from build123d import *

# Parameters (mm, degrees)
SKETCH1_R           = 1.4
BOSS_EXTRUDE1_DEPTH = 3
SKETCH2_R           = 1.4
BOSS_EXTRUDE2_DEPTH = 3
SKETCH3_W           = 32
SKETCH3_H           = 35.2
BOSS_EXTRUDE3_DEPTH = 3


with BuildPart() as part:
    # Sketch1 → Boss-Extrude1 (new body)
    with BuildSketch(Plane(origin=(0, 0, 0), x_dir=(1, 0, 0), z_dir=(0, 1, 0))):
        Polygon((-16, 24), (-16, -6), (16, -6), (16, 24), (10, 24), (10, 0), (-10, 0), (-10, 24), align=None)
        with Locations(Location((-8, -3.307692308, 0), (0, 0, 270))):
            Circle(SKETCH1_R, mode=Mode.SUBTRACT)
        with Locations(Location((8, -3.307692308, 0), (0, 0, 90))):
            Circle(SKETCH1_R, mode=Mode.SUBTRACT)
        with Locations(Location((-13.5, 18.192307692, 0), (0, 0, 270))):
            Circle(SKETCH1_R, mode=Mode.SUBTRACT)
        with Locations(Location((-13.5, 10.192307692, 0), (0, 0, 270))):
            Circle(SKETCH1_R, mode=Mode.SUBTRACT)
        with Locations(Location((-13.5, 2.192307692, 0), (0, 0, 270))):
            Circle(SKETCH1_R, mode=Mode.SUBTRACT)
        with Locations(Location((13.5, 2.192307692, 0), (0, 0, 90))):
            Circle(SKETCH1_R, mode=Mode.SUBTRACT)
        with Locations(Location((13.5, 10.192307692, 0), (0, 0, 90))):
            Circle(SKETCH1_R, mode=Mode.SUBTRACT)
        with Locations(Location((13.5, 18.192307692, 0), (0, 0, 90))):
            Circle(SKETCH1_R, mode=Mode.SUBTRACT)
    extrude(amount=BOSS_EXTRUDE1_DEPTH)



with BuildPart() as body_2:
    # Sketch2 → Boss-Extrude2 (new body)
    with BuildSketch(Plane(origin=(0, 32.2, 0), x_dir=(1, 0, 0), z_dir=(0, 1, 0))):
        Polygon((16, 24), (10, 24), (10, 0), (-10, 0), (-10, 24), (-16, 24), (-16, -6), (16, -6), align=None)
        with Locations(Location((-13.5, 18.192307692, 0), (0, 0, 270))):
            Circle(SKETCH2_R, mode=Mode.SUBTRACT)
        with Locations(Location((13.5, 18.192307692, 0), (0, 0, 90))):
            Circle(SKETCH2_R, mode=Mode.SUBTRACT)
        with Locations(Location((13.5, 10.192307692, 0), (0, 0, 90))):
            Circle(SKETCH2_R, mode=Mode.SUBTRACT)
        with Locations(Location((13.5, 2.192307692, 0), (0, 0, 90))):
            Circle(SKETCH2_R, mode=Mode.SUBTRACT)
        with Locations(Location((8, -3.307692308, 0), (0, 0, 90))):
            Circle(SKETCH2_R, mode=Mode.SUBTRACT)
        with Locations(Location((-8, -3.307692308, 0), (0, 0, 270))):
            Circle(SKETCH2_R, mode=Mode.SUBTRACT)
        with Locations(Location((-13.5, 10.192307692, 0), (0, 0, 270))):
            Circle(SKETCH2_R, mode=Mode.SUBTRACT)
        with Locations(Location((-13.5, 2.192307692, 0), (0, 0, 270))):
            Circle(SKETCH2_R, mode=Mode.SUBTRACT)
    extrude(amount=BOSS_EXTRUDE2_DEPTH)


with BuildPart() as part_1:
    add(part.part)

    add(body_2.part)  # Boss-Extrude3 merges body 2
    # Sketch3 → Boss-Extrude3 (add)
    with BuildSketch(Plane.XY.offset(6)):
        with Locations((0, 17.6)):
            Rectangle(SKETCH3_W, SKETCH3_H)
    extrude(amount=BOSS_EXTRUDE3_DEPTH)


solid = part_1.part
Design review of the part built by this model. Coordinates are the model's own, in mm. A direction names the side the tool comes from. Coordinates: 2 decimals unless noted, no trailing zeros. Loops run counter-clockwise (first coordinate to the right, second up) from the corner with the lowest first, then second, coordinate; pieces in that order, holes last. Notation, with made-up numbers: (28.5, 12.5) -> (39.5, 12.5) arc R19 cw to (39.5, 36.5) -> close; hole circle Ø2 at (7.25, 50.5). An arc over 180 degrees is marked (long way). Use a Markdown table: item, result. Add a question column.
Item 1: We need section C-C, the plane z = -2. Count the separate pieces of the cut face and the enclosed holes in it, and give its area (3 significant figures).
Item 2: Machinability: for faces 1 (the flat face through (0, 18, 6)), 2 (the flat face through (13, 34, -24)), 3 (the flat face through (-10, 34, -12)), which of the approach directions +Z, -Z, +X, -X, +Y, -Y give a long, thin tool a straight path to every point of the face, cutting with its end or side? Answer none if there is none.
Item 3: Clearance check with flat-ended pins moving along their axes: P1, Ø1.5, axis at x = -4, y = 34.5, coming from the -Z side; P2, Ø4.5, axis at x = 13.5, z = -10.19, coming from the +Y side; P3, Ø14.5, axis at x = 2.5, y = 22, coming from the -Z side. State where each tip first meets the part, or that it passes through.
Item 4: Wall thickness on L1, parallel to Z at x = 13.5, y = 32.95; L2, parallel to Y at x = 13, z = -20; L3, parallel to Z at x = -7.5, y = 6.5: over which ranges is each line inside the solid? List them lowest first. Write a range as from..to.
Item 5: We need section A-A, the plane z = -22. Write out the cut boundary in (x, y).
Item 6: The part is to be moulded in two halves that separate along X. For faces 4 (the cylindrical face through (-9.367, 1.479, 3.004)), 5 (the flat face through (0, 35.2, 3)), say which applies: +X half, -X half, draft (parallel to the pull), parting line (faces both ways), or undercut.
Item 7: We need section B-B, the plane x = 8. Write out the cut boundary in (y, z), and give its area (3 significant figures).
Numbers:
| question | item | result |
|---|---|---|
| 1 | separate pieces | 8 |
| 1 | enclosed holes | 0 |
| 1 | area | 38.7 mm^2 |
| 2 | face 1 | -Z, +X, -X |
| 2 | face 2 | -Z, +X, -X, +Y, -Y |
| 2 | face 3 | -Z, +Y, -Y |
| 3 | P1 | stops at z = 0 |
| 3 | P2 | stops at y = 35.2 |
| 3 | P3 | stops at z = 6 |
| 4 | L1 | z = -24..-19.59, -16.79..-11.59, -8.79..-3.59, -0.79..9 |
| 4 | L2 | y = 0..3, 32.2..35.2 |
| 4 | L3 | z = 6..9 |
| 5 | outline | (-16, 0) -> (-10, 0) -> (-10, 3) -> (-16, 3) -> close; (-16, 32.2) -> (-10, 32.2) -> (-10, 35.2) -> (-16, 35.2) -> close; (10, 0) -> (16, 0) -> (16, 3) -> (10, 3) -> close; (10, 32.2) -> (16, 32.2) -> (16, 35.2) -> (10, 35.2) -> close |
| 6 | face 4 | undercut |
| 6 | face 5 | draft |
| 7 | outline | (0, 0) -> (3, 0) -> (3, 1.91) -> (0, 1.91) -> close; (0, 4.71) -> (3, 4.71) -> (3, 6) -> (32.2, 6) -> (32.2, 4.71) -> (35.2, 4.71) -> (35.2, 9) -> (0, 9) -> close; (32.2, 0) -> (35.2, 0) -> (35.2, 1.91) -> (32.2, 1.91) -> close |
| 7 | area | 125 mm^2 |
